Part model, mm, in its own coordinate system. Round coordinates to 2 decimals unless told otherwise and drop trailing zeros. Write each loop counter-clockwise with the first axis right and the second up, starting at its lowest first coordinate (ties: lowest second). Pieces come first, ordered by that corner, then holes.
1) Saw through at A-A on y = -0.3. Write the cut outline in (x, z), and give its area (3 significant figures).
2) Drill centre lines: L1, parallel to X at y = -1.3, z = -0.05; L2, parallel to Z at x = -3, y = -0.85; L3, parallel to X at y = -1.7, z = 0.8. Where is each one in solid material? Low to high.
3) Pull direction X, two halves, no side cores. Call faces 1 (the flat face through (-2, 0, -2.5)), 2 (the cylindrical face through (-0.27, 0.03, 1.22)), 3 (the flat face through (-5.5, 0, -1)), 4 (the cylindrical face through (-1.81, 0.03, -0.38)): +X half, -X half, draft (parallel to the pull), parting line (faces both ways), or undercut.
4) Flat gauge pin, fed straight in: pin 1 (2 mm diameter, centred on x = -3, z = 0, fed in from -Y). Where does the tip first touch, or does it go through?
Solid Edge part; units mm, degrees
sketch "Sketch1" plane through (0, 0, 0) normal (0, -1, 0) x (1, 0, 0)
  circle A0 centre (0, 0) radius 1.25
  circle A1 centre (-3, 0) radius 1.25
  line L0 (-3, 2.5) -> (0, 2.5)
  line L1 (2.5, 0) -> (2.5, -2.5)
  line L2 (0, -2.5) -> (2.5, -2.5)
  line L3 (0, -2.5) -> (-3, -2.5)
  line L4 (-3, -2.5) -> (-5.5, -2.5)
  line L5 (-5.5, 0) -> (-5.5, -2.5)
  arc A2 (-5.5, 0) -> (-3, 2.5) centre (-3, 0) cw
  arc A3 (0, 2.5) -> (2.5, 0) centre (0, 0) cw
extrude "Protrusion1" add sketch "Sketch1" along normal mid plane 5
fillet "Verrundung_1" radius 0.5 10 edges at (-4.7678, -2.5, 1.7678) (-1.5, -2.5, 2.5) (1.7678, -2.5, 1.7678) (2.5, -2.5, -1.25) (-5.5, -2.5, -1.25) (-1.5, 2.5, 2.5) (1.7678, 2.5, 1.7678) (2.5, 2.5, -1.25) (-4.7678, 2.5, 1.7678) (-5.5, 2.5, -1.25)
chamfer "Fase_1" distance 0.25 angle 45 4 edges at (-4.25, -2.5, 0) (-1.25, -2.5, 0) (-4.25, 2.5, 0) (-1.25, 2.5, 0)
properties part number "085" material "PLA"
Completed:
1. outline: (-5.5, -2.5) - (2.5, -2.5) - (2.5, 0) arc R2.5 ccw to (0, 2.5) - (-3, 2.5) arc R2.5 ccw to (-5.5, 0) - close; hole circle Ø2.5 at (-3, 0); hole circle Ø2.5 at (0, 0)
1. area: 27.5 mm2
2. L1: x = -5.5 to -4.25, -1.75 to -1.25, 1.25 to 2.5
2. L2: z = -2.5 to -1.25, 1.25 to 2.5
2. L3: x = -5.37 to -3.96, -2.04 to -0.96, 0.96 to 2.37
3. face 1: draft
3. face 2: undercut
3. face 3: -X half
3. face 4: undercut
4. pin 1: passes through
